from build123d import *

# Parameters (mm, degrees)
BOSS_EXTRUDE1_DEPTH = 5
HOLE1_D             = 3
HOLE1_CBORE_D       = 5.5
HOLE1_CBORE_DEPTH   = 2.5
HOLE2_D             = 3
HOLE2_CBORE_D       = 5.5
HOLE2_CBORE_DEPTH   = 2.5
FILLET1_R           = 2


with BuildPart() as part:
    # Sketch2 → Boss-Extrude1 (new body)
    with BuildSketch(Plane.XY):
        Polygon((-31, 0), (-31, 28), (-16.5, 28), (-16.5, 108), (16.5, 108), (16.5, 28), (31, 28), (31, 0), align=None)
    extrude(amount=BOSS_EXTRUDE1_DEPTH)

    # Hole1 (through all)
    with Locations(Plane.XY.offset(5)):
        with Locations((-25.5, 5.5), (25.5, 5.5), (0, 23.5)):
            CounterBoreHole(HOLE1_D / 2, HOLE1_CBORE_D / 2, HOLE1_CBORE_DEPTH)

    # Hole2 (through all)
    with Locations(Plane(origin=(0, 0, 0), x_dir=(1, 0, 0), z_dir=(0, 0, -1))):
        with Locations((8, -48), (-8, -48), (-8, -88), (8, -88)):
            CounterBoreHole(HOLE2_D / 2, HOLE2_CBORE_D / 2, HOLE2_CBORE_DEPTH)

    # Fillet1
    fillet1_edges = [part.edges().sort_by_distance(p)[0] for p in [
        (-31, 0, 2.5),
        (-31, 28, 2.5),
        (-16.5, 108, 2.5),
        (16.5, 108, 2.5),
        (31, 28, 2.5),
        (31, 0, 2.5),
    ]]
    fillet(fillet1_edges, radius=FILLET1_R)


solid = part.part
The listing builds one solid part. Answer for the finished solid, in the listing's coordinates (mm). A direction names the side the tool comes from. Coordinates: 2 decimals unless noted, no trailing zeros. Write each loop counter-clockwise with the first axis right and the second up, starting at its lowest first coordinate (ties: lowest second). Pieces come first, ordered by that corner, then holes. Notation, with made-up numbers: M 19,-23 L 45,-23 A24 cw 45,-5 Z; hole C 63.5,41 d3. An arc over 180 degrees is marked long. Put each result on its own line as item: value. Start each with the question number.
1. For a pull along Y with two mould halves and no side action, classify faces 1 (the flat face through (-23, 28, 2)), 2 (the cylindrical face through (30.4, 0.57, 2.54)), 3 (the flat face through (-24, 4, 2.5)), 4 (the flat face through (-31, 14, 2)) as pulls with the +Y half, pulls with the -Y half, needs draft (parallel to the pull), parting line crosses it, or undercut.
2. Which of the six approach directions +Z, -Z, +X, -X, +Y, -Y give full straight-line access (tool end or side, diameter ignored) to faces 5 (the cylindrical face through (8.325, 49.464, 3.768)), 6 (the flat face through (-16.5, 66, 2)), 7 (the cylindrical face through (-8.358, 45.273, 1.232))?
3. A cutting plane is placed at C-C on x = -8. Write down the section's boundary in (y, z), then the cut area to 4 significant figures.
4. A cutting plane is placed at A-A on y = 5.5. Write down the section's boundary in (x, z).
5. A cutting plane is placed at B-B on x = 0. Write down the section's boundary in (y, z), then the cut area to 3 significant figures.
6. Consider line 1 (X direction, y = 88, z = 1.5); line 2 (X direction, y = 48, z = 3.25); line 3 (Y direction, x = -8, z = 1.6). Determine where each line is inside the solid, lowest interval first. Write a range as from..to.
7. A cutting plane is placed at D-D on y = 23.5. Write down the section's boundary in (x, z).
8. Flat-ended cylindrical pins translate along their axes: P1, Ø2.5, axis at x = -8, y = 48, coming from the +Z side; P2, Ø3, axis at x = 9, y = 48, coming from the -Z side; P3, Ø5, axis at x = -25.5, y = 5.5, coming from the +Z side. Find the tip coordinate at first contact, or state that the pin passes through.
Resolved:
1. face 1: pulls with the +Y half
1. face 2: pulls with the -Y half
1. face 3: undercut
1. face 4: needs draft
2. face 5: +Z, -Z
2. face 6: +Z, -Z, -X, +Y
2. face 7: -Z
3. outline: M 0,0 L 45.25,0 L 45.25,2.5 L 46.5,2.5 L 46.5,5 L 0,5 Z; M 49.5,2.5 L 50.75,2.5 L 50.75,0 L 85.25,0 L 85.25,2.5 L 86.5,2.5 L 86.5,5 L 49.5,5 Z; M 89.5,2.5 L 90.75,2.5 L 90.75,0 L 108,0 L 108,5 L 89.5,5 Z
3. area: 497.5 mm2
4. outline: M -31,0 L -27,0 L -27,2.5 L -28.25,2.5 L -28.25,5 L -31,5 Z; M -24,0 L 24,0 L 24,2.5 L 22.75,2.5 L 22.75,5 L -22.75,5 L -22.75,2.5 L -24,2.5 Z; M 27,0 L 31,0 L 31,5 L 28.25,5 L 28.25,2.5 L 27,2.5 Z
5. outline: M 0,0 L 22,0 L 22,2.5 L 20.75,2.5 L 20.75,5 L 0,5 Z; M 25,0 L 108,0 L 108,5 L 26.25,5 L 26.25,2.5 L 25,2.5 Z
5. area: 519 mm2
6. line 1: x = -16.5..-10.75, -5.25..5.25, 10.75..16.5
6. line 2: x = -16.5..-9.5, -6.5..6.5, 9.5..16.5
6. line 3: y = 0..45.25, 50.75..85.25, 90.75..108
7. outline: M -31,0 L -1.5,0 L -1.5,2.5 L -2.75,2.5 L -2.75,5 L -31,5 Z; M 1.5,0 L 31,0 L 31,5 L 2.75,5 L 2.75,2.5 L 1.5,2.5 Z
8. P1: passes through
8. P2: stops at z = 2.5
8. P3: stops at z = 2.5
